```python
from build123d import *

# Parameters (mm, degrees)
SKETCH1_R           = 2.1
BOSS_EXTRUDE1_DEPTH = 25
SKETCH2_W           = 203.2
SKETCH2_H           = 203.2
BOSS_EXTRUDE2_DEPTH = 1.5
SKETCH3_R           = 10
BOSS_EXTRUDE3_DEPTH = 1


with BuildPart() as part:
    # Sketch1 → Boss-Extrude1 (new body)
    with BuildSketch(Plane(origin=(0, 0, 0), x_dir=(1, 0, 0), z_dir=(0, 1, 0))):
        with Locations(Location((0, 0, 0), (0, 0, 270))):
            Circle(SKETCH1_R)
    extrude(amount=-BOSS_EXTRUDE1_DEPTH)

    # Sketch2 → Boss-Extrude2 (add)
    with BuildSketch(Plane(origin=(0, 0, 0), x_dir=(1, 0, 0), z_dir=(0, 1, 0))):
        Rectangle(SKETCH2_W, SKETCH2_H)
    extrude(amount=BOSS_EXTRUDE2_DEPTH)

    # Sketch3 → Boss-Extrude3 (add)
    with BuildSketch(Plane(origin=(0, 0, 0), x_dir=(1, 0, 0), z_dir=(0, 1, 0))):
        with Locations(Location((0, 0, 0), (0, 0, 270))):
            Circle(SKETCH3_R)
    extrude(amount=-BOSS_EXTRUDE3_DEPTH)


solid = part.part
```
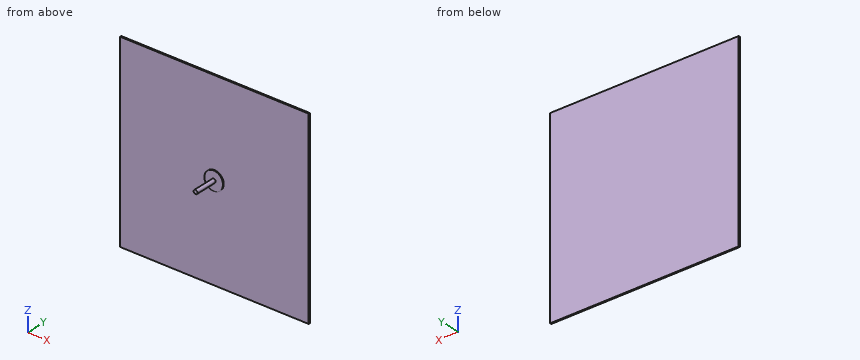
Here's how the part is built. I have some questions about the finished solid (model axes, mm). Give positions to 0.01 mm unless a question says otherwise; leave off trailing zeros. Loops run counter-clockwise (first coordinate to the right, second up) from the corner with the lowest first, then second, coordinate; pieces in that order, holes last. Notation, with made-up numbers: M 53.5,68.25 L 62.5,68.25 A29 cw 62.5,94.25 Z; hole C -39,68 d11. An arc over 180 degrees is marked long. Put each result on its own line as item: value. Start each with the question number.
(1) I want a section at B-B on y = -11.75. Please give me the cut outline in (x, z).
(2) Will these pins go through, and if not, where does the flat tip stop? pin 1 Ø1 at (x, z) = (38.5, -81) entering from -Y; pin 2 Ø1.5 at (y, z) = (-1.5, 0.5) entering from -X.
(3) I need wall thicknesses on line 1 along Y through (x, z) = (-84, 43.5). Which ranges of the line are inside material? Lowest first, please. Write a range as [from, to].
(4) I want a section at A-A on z = -30. Please give me the cut outline in (x, y).
(5) I want a section at C-C on z = 7. Please give me the cut outline in (x, y).
Answer block:
1. outline: C 0,0 d4.2
2. pin 1: y = 0
2. pin 2: x = -10
3. line 1: [0, 1.5]
4. outline: M -101.6,0 L 101.6,0 L 101.6,1.5 L -101.6,1.5 Z
5. outline: M -101.6,0 L -7.14,0 L -7.14,-1 L 7.14,-1 L 7.14,0 L 101.6,0 L 101.6,1.5 L -101.6,1.5 Z
